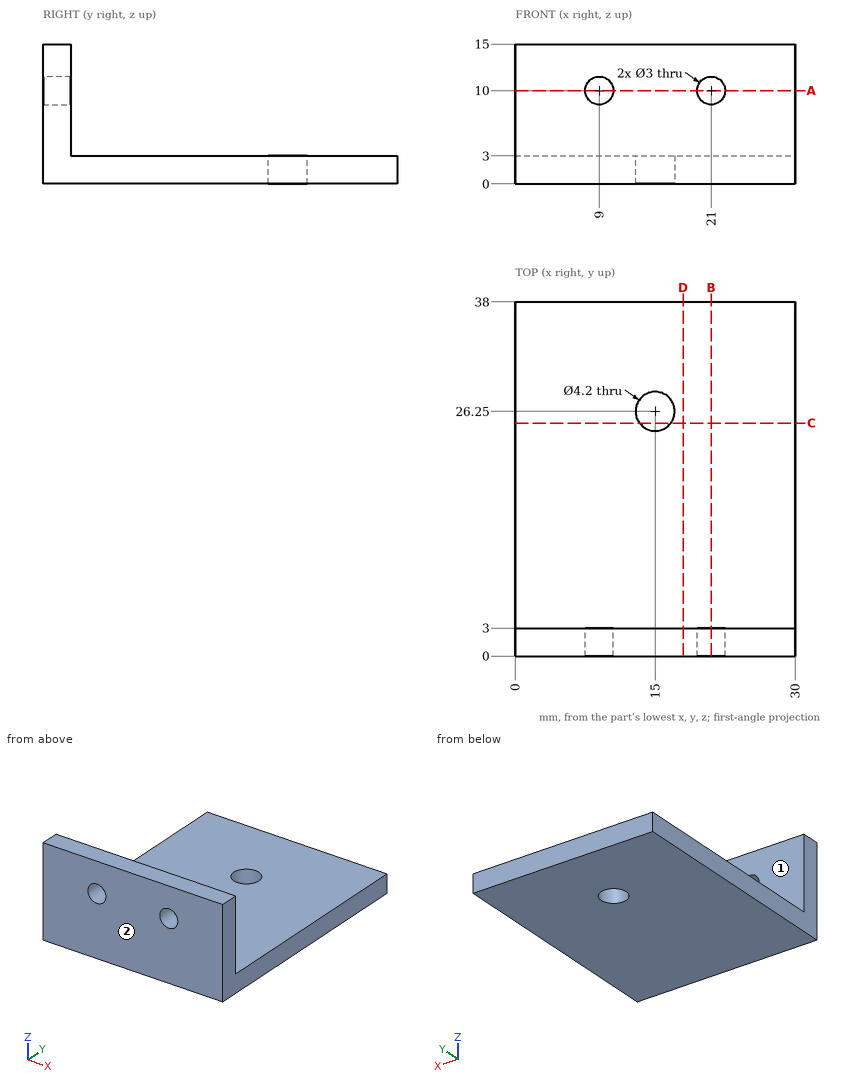
Check sheet for the drawn part. Datum: minimum x, y, z corner. Units: mm. A direction names the side the tool comes from. Round coordinates to 2 decimals unless told otherwise and drop trailing zeros. Order: outer loops, then holes, each group sorted by start corner. A loop starts at its lowest first (then second) coordinate and runs counter-clockwise, first axis right, second up. Notation, with made-up numbers: (37, 75) -> (77, 75) arc R29 cw to (77, 103) -> close; hole circle Ø1 at (75.25, 17.25). An arc over 180 degrees is marked (long way). Put each result on its own line as item: value. Start each with the question number.
(1) Depth check by flat-ended pin: pin 1 Ø5 at (x, z) = (12.5, 9) entering from +Y; pin 2 Ø15 at (x, y) = (12.5, 15) entering from +Z. Enter the tip coordinate at first touch or a pass-through.
(2) Tool access check on the marked faces 1 and 2. Record the directions out of +Z, -Z, +X, -X, +Y, -Y that give a thin tool (end or side, any length) a straight path to the whole face; none if there is none.
(3) Material ranges on line 1 along Y through (x, z) = (15, 1.15); line 2 along Y through (x, z) = (22.25, 4.75), recorded low to high.
(4) Section check B-B (x = 21). Enter the section's corners in (y, z), then the cut area to 3 significant figures.
(5) Section check D-D (x = 18). Enter the section's corners in (y, z).
(6) Section check C-C (y = 25). Enter the section's corners in (x, z).
(7) Section check A-A (z = 10). Enter the section's corners in (x, y).
Completed:
1. pin 1: stops at y = 3
1. pin 2: stops at z = 3
2. face 1: +Z, +X, -X, +Y
2. face 2: +Z, -Z, +X, -X, -Y
3. line 1: y = 0 to 24.15, 28.35 to 38
3. line 2: y = 0 to 3
4. outline: (0, 0) -> (38, 0) -> (38, 3) -> (3, 3) -> (3, 8.5) -> (0, 8.5) -> close; (0, 11.5) -> (3, 11.5) -> (3, 15) -> (0, 15) -> close
4. area: 141 mm2
5. outline: (0, 0) -> (38, 0) -> (38, 3) -> (3, 3) -> (3, 15) -> (0, 15) -> close
6. outline: (0, 0) -> (13.31, 0) -> (13.31, 3) -> (0, 3) -> close; (16.69, 0) -> (30, 0) -> (30, 3) -> (16.69, 3) -> close
7. outline: (0, 0) -> (7.5, 0) -> (7.5, 3) -> (0, 3) -> close; (10.5, 0) -> (19.5, 0) -> (19.5, 3) -> (10.5, 3) -> close; (22.5, 0) -> (30, 0) -> (30, 3) -> (22.5, 3) -> close
